Geometry check sheet. Reference: drawing and pictorial views, mm from the part's lowest x, y, z. Round coordinates to 2 decimals unless told otherwise and drop trailing zeros. Write each loop counter-clockwise with the first axis right and the second up, starting at its lowest first coordinate (ties: lowest second). Pieces come first, ordered by that corner, then holes. Notation, with made-up numbers: M -23.75,-0.5 L 25.25,-0.5 A17 ccw 25.25,16.5 Z; hole C 3,52.25 d2. An arc over 180 degrees is marked long. One line per item, written item: value. Start each with the question number.
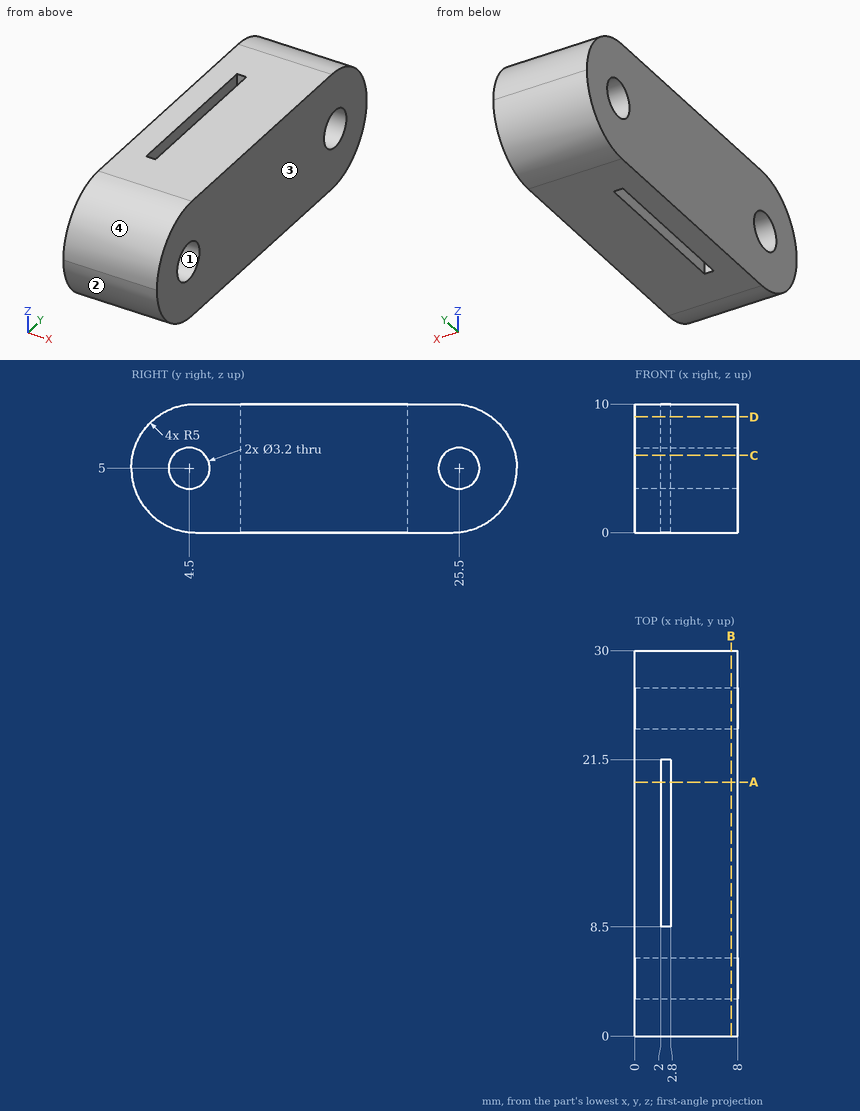
1) Gauge pin test, flat ends, axial feed: pin 1 Ø0.6 at (x, z) = (2.5, 4) entering from +Y; pin 2 Ø1.5 at (x, z) = (1, 3) entering from +Y; pin 3 Ø2 at (x, z) = (2.5, 3.5) entering from -Y (3 decimals). Record the tip position at first contact, or that the pin passes through.
2) Cross-section at A-A (y = 19.75). Record the boundary of the cut face in (x, z), then the cut area to 3 significant figures.
3) Mould release check, pull along Z, two halves, no side actions. Record for the marked faces 1, 2, 3 and 4: pulls with the +Z half, pulls with the -Z half, needs draft (parallel to the pull), parting line crosses it, or undercut.
4) Cross-section at D-D (z = 9). Record the boundary of the cut face in (x, y).
5) Cross-section at B-B (x = 7.5). State how many separate pieces and enclosed holes the cut face has, then the cut area to 3 significant figures.
6) Cross-section at C-C (z = 6). Record the boundary of the cut face in (x, y), then the cut area to 3 significant figures.
7) Thickness scan on line 1 (Y direction, x = 2.75, z = 5); line 2 (Y direction, x = 5.5, z = 5); line 3 (X direction, y = 13, z = 6). Record the ranges inside material, lowest first.
Results below:
1. pin 1: stops at y = 29.95
1. pin 2: stops at y = 29.84
1. pin 3: stops at y = 0.025
2. outline: M 0,0 L 2,0 L 2,10 L 0,10 Z; M 2.8,0 L 8,0 L 8,10 L 2.8,10 Z
2. area: 72.0 mm²
3. face 1: undercut
3. face 2: pulls with the -Z half
3. face 3: needs draft
3. face 4: pulls with the +Z half
4. outline: M 0,2 L 8,2 L 8,28 L 0,28 Z; hole M 2,8.5 L 2.8,8.5 L 2.8,21.5 L 2,21.5 Z
5. separate pieces: 1
5. enclosed holes: 2
5. area: 262 mm²
6. outline: M 0,0.1 L 8,0.1 L 8,3.25 L 0,3.25 Z; M 0,5.75 L 8,5.75 L 8,24.25 L 0,24.25 Z; M 0,26.75 L 8,26.75 L 8,29.9 L 0,29.9 Z; hole M 2,8.5 L 2.8,8.5 L 2.8,21.5 L 2,21.5 Z
6. area: 188 mm²
7. line 1: y = 0 to 2.9, 6.1 to 8.5, 21.5 to 23.9, 27.1 to 30
7. line 2: y = 0 to 2.9, 6.1 to 23.9, 27.1 to 30
7. line 3: x = 0 to 2, 2.8 to 8
